```python
from build123d import *

# Parameters (mm, degrees)
F1_DEPTH = 5
F2_DEPTH = 1.5
F3_R     = 1.5
F4_DEPTH = 3.001


with BuildPart() as f1:
    # F0 (on Front) → F1 (new body, symmetric)
    with BuildSketch(Plane.XZ):
        Polygon((5, -1.5), (10, -1.5), (10, 1.5), (-10, 1.5), (-10, -1.5), (-5, -1.5), (0, -1.5), align=None)
    extrude(amount=F1_DEPTH, both=True)

    # F0 (on Front) → F2 (join, symmetric)
    with BuildSketch(Plane.XZ):
        Polygon((5, -1.5), (10, -1.5), (10, 1.5), (-10, 1.5), (-10, -1.5), (-5, -1.5), (0, -1.5), align=None)
        with BuildLine():
            Line((5, -8.5), (5, -1.5))
            Line((5, -1.5), (0, -1.5))
            Line((0, -1.5), (-5, -1.5))
            Line((-5, -1.5), (-5, -8.5))
            Line((-5, -8.5), (-1.75, -8.5))
            ThreePointArc((-1.75, -8.5), (0, -6.75), (1.75, -8.5))
            Line((1.75, -8.5), (5, -8.5))
        make_face()
        with BuildLine():
            ThreePointArc((-5, -8.5), (0, -13.5), (5, -8.5))
            Line((5, -8.5), (1.75, -8.5))
            ThreePointArc((1.75, -8.5), (0, -10.25), (-1.75, -8.5))
            Line((-1.75, -8.5), (-5, -8.5))
        make_face()
    extrude(amount=F2_DEPTH, both=True)

    # F3 (on face) → F4 (cut, through all)
    with BuildSketch(Plane(origin=(0, 0, -1.5), x_dir=(1, 0, 0), z_dir=(0, 0, -1))):
        with Locations((-7, 0)):
            Circle(F3_R)
        with Locations((7, 0)):
            Circle(F3_R)
    extrude(amount=-F4_DEPTH, mode=Mode.SUBTRACT)


solid = f1.part
```
For this review, take the finished solid that the model builds, in its own axes (mm). A direction names the side the tool comes from. Coordinates: 2 decimals unless noted, no trailing zeros. Loops run counter-clockwise (first coordinate to the right, second up) from the corner with the lowest first, then second, coordinate; pieces in that order, holes last. Notation, with made-up numbers: (-21, 58) -> (30, 58) arc R32 ccw to (30, 92) -> close; hole circle Ø5 at (-30.5, -8.75). An arc over 180 degrees is marked (long way). Return JSON: item names as keys, results as strings. Group by question number.
(1) Consider section B-B, the plane y = -0.75. Give the boundary of the cut face in (x, z), plus the area to 3 significant figures.
(2) Tool access review of faces 5 (the flat face through (0, 1.5, -6)), 6 (the flat face through (5, 0, -5)), 7 (the flat face through (0, -1.5, -6)): name each direction out of +Z, -Z, +X, -X, +Y, -Y from which nothing blocks a thin tool from reaching the whole face with its end or side.
(3) Consider section C-C, the plane z = -7.25. Give the boundary of the cut face in (x, y), plus the area to 3 significant figures.
(4) Consider section A-A, the plane x = -7. Give the boundary of the cut face in (y, z), plus the area to 3 significant figures.
(5) For pin 1 Ø3 at (y, z) = (-2.5, -8) entering from +X; pin 2 Ø3 at (x, z) = (6.5, -11) entering from +Y; pin 3 Ø1 at (x, y) = (-6.5, -3.5) entering from -Z; pin 4 Ø5 at (x, z) = (-2.5, -7) entering from -Y, all flat-tipped, find the tip position at first contact; note any pin that passes through.
(6) To check wall thickness, follow L1, parallel to X at y = 0, z = 0.3; L2, parallel to Y at x = -7, z = -0.8; L3, parallel to X at y = 0.8, z = -8.5. State the ranges of each line that lie inside material, in increasing order.
(7) Consider section D-D, the plane x = 0. Give the boundary of the cut face in (y, z), plus the area to 3 significant figures.
(8) Mouldability with a two-part tool opening along X and no side actions: class faces 1 (the flat face through (0, 5, 0)), 2 (the cylindrical face through (-0.228, -0.021, -10.235)), 3 (the cylindrical face through (5.5, -0.07, -0.02)), 4 (the flat face through (-10, 0, 0)) as pulls with the +X half, pulls with the -X half, needs draft (parallel to the pull), parting line crosses it, or undercut.
Results below:
{
 "1": {"outline": "(-10, -1.5) -> (-8.3, -1.5) -> (-8.3, 1.5) -> (-10, 1.5) -> close; (-5.7, -1.5) -> (-5, -1.5) -> (-5, -8.5) arc R5 ccw to (5, -8.5) -> (5, -1.5) -> (5.7, -1.5) -> (5.7, 1.5) -> (-5.7, 1.5) -> close; (8.3, -1.5) -> (10, -1.5) -> (10, 1.5) -> (8.3, 1.5) -> close; hole circle Ø3.5 at (0, -8.5)", "area": "144 mm2"},
 "2": {"face 5": "-Z, +X, -X, +Y", "face 6": "-Z, +X, +Y, -Y", "face 7": "-Z, +X, -X, -Y"},
 "3": {"outline": "(-5, -1.5) -> (-1.22, -1.5) -> (-1.22, 1.5) -> (-5, 1.5) -> close; (1.22, -1.5) -> (5, -1.5) -> (5, 1.5) -> (1.22, 1.5) -> close", "area": "22.7 mm2"},
 "4": {"outline": "(-5, -1.5) -> (-1.5, -1.5) -> (-1.5, 1.5) -> (-5, 1.5) -> close; (1.5, -1.5) -> (5, -1.5) -> (5, 1.5) -> (1.5, 1.5) -> close", "area": "21.0 mm2"},
 "5": {"pin 1": "stops at x = 5", "pin 2": "passes through", "pin 3": "stops at z = -1.5", "pin 4": "stops at y = -1.5"},
 "6": {"L1": "x = -10 to -8.5, -5.5 to 5.5, 8.5 to 10", "L2": "y = -5 to -1.5, 1.5 to 5", "L3": "x = -5 to -1.75, 1.75 to 5"},
 "7": {"outline": "(-5, -1.5) -> (-1.5, -1.5) -> (-1.5, -6.75) -> (1.5, -6.75) -> (1.5, -1.5) -> (5, -1.5) -> (5, 1.5) -> (-5, 1.5) -> close; (-1.5, -13.5) -> (1.5, -13.5) -> (1.5, -10.25) -> (-1.5, -10.25) -> close", "area": "55.5 mm2"},
 "8": {"face 1": "needs draft", "face 2": "undercut", "face 3": "undercut", "face 4": "pulls with the -X half"}
}
